from build123d import *

# Parameters (mm, degrees)
EXTRUDE_1_DEPTH     = 8
EXTRUDE_2_DEPTH     = 5
SKETCH_4_R          = 16.5
CUT_EXTRUDE_1_DEPTH = 3
SKETCH_5_R          = 13
EXTRUDE_3_DEPTH     = 4.5
SKETCH_6_R          = 6
CUT_EXTRUDE_3_DEPTH = 53.834647723
FILLET_1_R          = 4
SKETCH_7_R          = 5
CUT_EXTRUDE_4_DEPTH = 2
CUT_EXTRUDE_5_REACH = 53.444
SKETCH_8_R          = 3.5


with BuildPart() as part:
    # 草图1 → 凸台-拉伸1 (new, symmetric)
    with BuildSketch(Plane.XY):
        with BuildLine():
            ThreePointArc((-16.322626067, 6.275192635), (0, -3), (16.322626067, 6.275192635))
            Line((16.322626067, 6.275192635), (17, -3))
            Line((17, -3), (35.5, -3))
            Line((35.5, -3), (35.5, 3))
            Line((35.5, 3), (20, 3))
            Line((20, 3), (18.949533673, 17.383897959))
            ThreePointArc((18.949533673, 17.383897959), (0, 35), (-18.949533673, 17.383897959))
            Line((-18.949533673, 17.383897959), (-20, 3))
            Line((-20, 3), (-35.5, 3))
            Line((-35.5, 3), (-35.5, -3))
            Line((-35.5, -3), (-17, -3))
            Line((-17, -3), (-16.322626067, 6.275192635))
        make_face()
    extrude(amount=EXTRUDE_1_DEPTH, both=True)

    # 草图3 → 凸台-拉伸2 (add, symmetric)
    with BuildSketch(Plane.XY):
        with BuildLine():
            Line((-16.322626067, 6.275192635), (-17, -3))
            Line((-17, -3), (-6e-08, -3))
            ThreePointArc((-6e-08, -3), (-9.386923379, -0.519251481), (-16.322626067, 6.275192635))
        make_face()
        with BuildLine():
            ThreePointArc((16.322626067, 6.275192635), (9.386923327, -0.51925151), (-6e-08, -3))
            Line((-6e-08, -3), (17, -3))
            Line((17, -3), (16.322626067, 6.275192635))
        make_face()
    extrude(amount=EXTRUDE_2_DEPTH, both=True)

    # 草图4 → 切除-拉伸1 (cut)
    with BuildSketch(Plane.XY.offset(8)):
        with Locations((0, 16)):
            Circle(SKETCH_4_R)
    cut_extrude_1 = extrude(amount=-CUT_EXTRUDE_1_DEPTH, mode=Mode.SUBTRACT)

    # 镜向1: 切除-拉伸1 across plane
    add(cut_extrude_1.mirror(Plane.XY), mode=Mode.SUBTRACT)

    # 草图5 → 凸台-拉伸3 (add)
    with BuildSketch(Plane.XY.offset(5)):
        with Locations(Location((0, 16, 0), (0, 0, 180))):
            Circle(SKETCH_5_R)
    extrude(amount=EXTRUDE_3_DEPTH)

    # 草图6 → 切除-拉伸3 (cut, through all)
    with BuildSketch(Plane.XY.offset(9.5)):
        with Locations((0, 16)):
            Circle(SKETCH_6_R)
    extrude(amount=-CUT_EXTRUDE_3_DEPTH, mode=Mode.SUBTRACT)

    # 圆角1
    fillet_1_edges = [part.edges().sort_by_distance(p)[0] for p in [
        (-35.5, 0, -8),
        (35.5, 0, -8),
        (35.5, 0, 8),
        (-35.5, 0, 8),
    ]]
    fillet(fillet_1_edges, radius=FILLET_1_R)

    # 草图7 → 切除-拉伸4 (cut)
    with BuildSketch(Plane.XZ.offset(3)):
        with Locations(Location((-28, 0, 0), (0, 0, 270))):
            Circle(SKETCH_7_R)
    cut_extrude_4 = extrude(amount=-CUT_EXTRUDE_4_DEPTH, mode=Mode.SUBTRACT)

    # 草图8 → 切除-拉伸5 (cut, up to next)
    with BuildSketch(Plane.XZ.offset(1), mode=Mode.PRIVATE) as cut_extrude_5_sk1:
        with Locations(Location((-28, 0, 0), (0, 0, 270))):
            Circle(SKETCH_8_R)
    cut_extrude_5_tool1 = extrude(cut_extrude_5_sk1.sketch, amount=-CUT_EXTRUDE_5_REACH, mode=Mode.PRIVATE) & part.part
    cut_extrude_5 = cut_extrude_5_tool1.solids().sort_by_distance((-28, -1, 0))[0]
    add(cut_extrude_5, mode=Mode.SUBTRACT)

    # 镜向2: 切除-拉伸4, 切除-拉伸5 across plane
    add(cut_extrude_4.mirror(Plane(origin=(0, 0, 0), x_dir=(0, 0, 1), z_dir=(1, 0, 0))), mode=Mode.SUBTRACT)
    add(cut_extrude_5.mirror(Plane(origin=(0, 0, 0), x_dir=(0, 0, 1), z_dir=(1, 0, 0))), mode=Mode.SUBTRACT)


solid = part.part
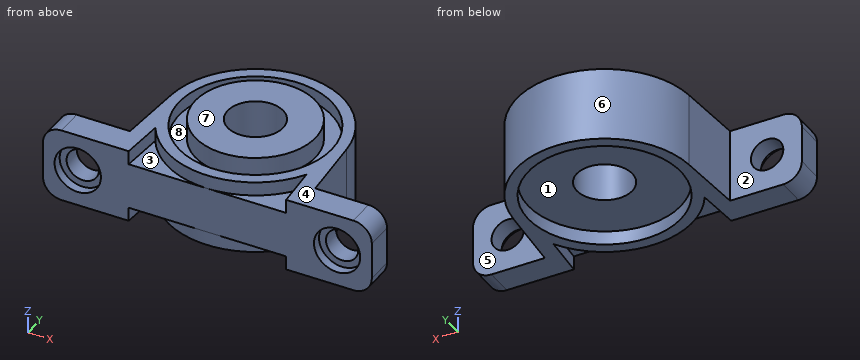
CAD build for the part. Positions are in the model's coordinates, mm. Face numbers are marked on the shaded views. A direction names the side the tool comes from. Coordinates: 2 decimals unless noted, no trailing zeros. Order: outer loops, then holes, each group sorted by start corner. A loop starts at its lowest first (then second) coordinate and runs counter-clockwise, first axis right, second up. Notation, with made-up numbers: (-30, 78.5) -> (-7, 78.5) arc R20 ccw to (-7, 108.5) -> close; hole circle Ø10 at (-39, 14.5). An arc over 180 degrees is marked (long way). Answer in a Markdown table with one row per item.
1) Drill centre lines: line 1 (X direction, y = -1.9, z = 0); line 2 (X direction, y = 0.2, z = 0); line 3 (Z direction, x = 28, y = 1.25). Where is each one in solid material? Low to high.
Check values:
| item | result |
|---|---|
| line 1 | -35.5 to -33, -23 to 23, 33 to 35.5 |
| line 2 | -35.5 to -31.5, -24.5 to 24.5, 31.5 to 35.5 |
| line 3 | -8 to -3.5, 3.5 to 8 |
2) Flat gauge pins, fed straight in: P1, Ø10, axis at y = 27, z = 3.5, coming from the +X side; P2, Ø5, axis at y = 24.5, z = 7.5, coming from the -X side; P3, Ø3, axis at x = -28, z = 1.5, coming from the -Y side; P4, Ø4, axis at x = 6.5, z = 4.5, coming from the +Y side. Where does each tip first touch, or does it go through?
Check values:
| item | result |
|---|---|
| P1 | x = 18.03 |
| P2 | x = -18.03 |
| P3 | through |
| P4 | y = 34.46 |
3) Mould opens along X. For the marked faces 6, 7 and 8 say: pulls with the +X half, pulls with the -X half, needs draft (parallel to the pull), parting line crosses it, or undercut.
Check values:
| item | result |
|---|---|
| face 6 | parting line crosses it |
| face 7 | needs draft |
| face 8 | undercut |
4) Band-saw the part on B-B (x = 28). List the corners of the cut face in (y, z).
Check values:
| item | result |
|---|---|
| outline | (-3, -8) -> (3, -8) -> (3, -3.5) -> (-1, -3.5) -> (-1, -5) -> (-3, -5) -> close; (-3, 5) -> (-1, 5) -> (-1, 3.5) -> (3, 3.5) -> (3, 8) -> (-3, 8) -> close |
5) Band-saw the part on A-A (z = 0). List the corners of the cut face in (x, y).
Check values:
| item | result |
|---|---|
| outline | (-35.5, -3) -> (-33, -3) -> (-33, -1) -> (-31.5, -1) -> (-31.5, 3) -> (-35.5, 3) -> close; (-24.5, -1) -> (-23, -1) -> (-23, -3) -> (23, -3) -> (23, -1) -> (24.5, -1) -> (24.5, 3) -> (20, 3) -> (18.95, 17.38) arc R19 ccw to (-18.95, 17.38) -> (-20, 3) -> (-24.5, 3) -> close; (31.5, -1) -> (33, -1) -> (33, -3) -> (35.5, -3) -> (35.5, 3) -> (31.5, 3) -> close; hole circle Ø12 at (0, 16) |
6) Band-saw the part on D-D (z = -6.5). List the corners of the cut face in (x, y).
Check values:
| item | result |
|---|---|
| outline | (-34.62, -3) -> (-17, -3) -> (-16.32, 6.28) arc R19 ccw to (16.32, 6.28) -> (17, -3) -> (34.62, -3) -> (34.62, 3) -> (20, 3) -> (18.95, 17.38) arc R19 ccw to (-18.95, 17.38) -> (-20, 3) -> (-34.62, 3) -> close; hole circle Ø33 at (0, 16) |
7) Band-saw the part on C-C (y = 12). List the corners of the cut face in (x, z).
Check values:
| item | result |
|---|---|
| outline | (-19.34, -8) -> (-16.01, -8) -> (-16.01, -5) -> (-4.47, -5) -> (-4.47, 9.5) -> (-12.37, 9.5) -> (-12.37, 5) -> (-16.01, 5) -> (-16.01, 8) -> (-19.34, 8) -> close; (4.47, -5) -> (16.01, -5) -> (16.01, -8) -> (19.34, -8) -> (19.34, 8) -> (16.01, 8) -> (16.01, 5) -> (12.37, 5) -> (12.37, 9.5) -> (4.47, 9.5) -> close |
8) Which spindle directions (+Z, -Z, +X, -X, +Y, -Y) get a long thin tool onto all of the face, cutting with end or side? Do the marked faces 1, 2, 3, 4 and 5. Say none if no direction does.
Check values:
| item | result |
|---|---|
| face 1 | -Z |
| face 2 | +Z, -Z, -X, +Y |
| face 3 | +Z, -Y |
| face 4 | +Z |
| face 5 | +Z, -Z, +X, +Y |
